from build123d import *

# Parameters (mm, degrees)
SKETCH1_R                = 2.55
BOSS_EXTRUDE1_DEPTH      = 5
SKETCH4_R                = 4.5
CUT_EXTRUDE2_DEPTH       = 1
SKETCH6_W                = 5.947651005
SKETCH6_H                = 20
BOSS_EXTRUDE2_DEPTH      = 4
BOSS_EXTRUDE2_DEPTH_BACK = 4
SKETCH11_R               = 4.5
CUT_EXTRUDE3_DEPTH       = 0.5
SKETCH16_R               = 3.25
BOSS_EXTRUDE3_DEPTH      = 3
BOSS_EXTRUDE3_DEPTH_BACK = 3
FILLET3_R                = 2
BOSS_EXTRUDE4_DEPTH      = 5.947651
CUT_EXTRUDE5_REACH       = 85
SKETCH18_R               = 3.25


with BuildPart() as part:
    # Sketch1 → Boss-Extrude1 (new body)
    with BuildSketch(Plane.XY):
        with BuildLine():
            Line((100, 25), (100, 20))
            ThreePointArc((100, 20), (99.414213562, 18.585786438), (98, 18))
            Line((98, 18), (72.248595461, 18))
            ThreePointArc((72.248595461, 18), (71.130561473, 17.658312395), (70.39454584, 16.75))
            ThreePointArc((70.39454584, 16.75), (50, 3), (29.60545416, 16.75))
            ThreePointArc((29.60545416, 16.75), (28.869438527, 17.658312395), (27.751404539, 18))
            Line((27.751404539, 18), (2, 18))
            ThreePointArc((2, 18), (0.585786438, 18.585786438), (0, 20))
            Line((0, 20), (0, 25))
            Line((0, 25), (0, 30))
            ThreePointArc((0, 30), (0.585786438, 31.414213562), (2, 32))
            Line((2, 32), (21.056240945, 32))
            Line((21.056240945, 32), (27.751404539, 32))
            ThreePointArc((27.751404539, 32), (28.869438527, 32.341687605), (29.60545416, 33.25))
            ThreePointArc((29.60545416, 33.25), (30.166752838, 34.520625347), (30.807119991, 35.753295167))
            ThreePointArc((30.807119991, 35.753295167), (32.106461975, 36.725482012), (33.699080137, 36.414026968))
            Line((33.699080137, 36.414026968), (35.34656276, 35.260447216))
            ThreePointArc((35.34656276, 35.260447216), (36.146649881, 34.078494315), (35.955031011, 32.664127224))
            ThreePointArc((35.955031011, 32.664127224), (50, 9), (64.044968989, 32.664127224))
            ThreePointArc((64.044968989, 32.664127224), (63.853350119, 34.078494315), (64.65343724, 35.260447216))
            Line((64.65343724, 35.260447216), (66.300919863, 36.414026968))
            ThreePointArc((66.300919863, 36.414026968), (67.893538025, 36.725482012), (69.192880009, 35.753295167))
            ThreePointArc((69.192880009, 35.753295167), (69.833247162, 34.520625347), (70.39454584, 33.25))
            ThreePointArc((70.39454584, 33.25), (71.130561473, 32.341687605), (72.248595461, 32))
            Line((72.248595461, 32), (78.943759055, 32))
            Line((78.943759055, 32), (98, 32))
            ThreePointArc((98, 32), (99.414213562, 31.414213562), (100, 30))
            Line((100, 30), (100, 25))
        make_face()
        with Locations((93, 25)):
            Circle(SKETCH1_R, mode=Mode.SUBTRACT)
        with Locations((7, 25)):
            Circle(SKETCH1_R, mode=Mode.SUBTRACT)
    extrude(amount=BOSS_EXTRUDE1_DEPTH)

    # Sketch4 → Cut-Extrude2 (cut)
    with BuildSketch(Plane.XY.offset(5)):
        with Locations((93, 25)):
            Circle(SKETCH4_R)
        with Locations((7, 25)):
            Circle(SKETCH4_R)
    extrude(amount=-CUT_EXTRUDE2_DEPTH, mode=Mode.SUBTRACT)

    # Sketch6 → Boss-Extrude2 (add, two sides)
    with BuildSketch(Plane(origin=(0, 25, 0), x_dir=(-1, 0, 0), z_dir=(0, -1, 0))) as boss_extrude2_sk:
        with Locations((-80.026174497, -15)):
            Rectangle(SKETCH6_W, SKETCH6_H)
    extrude(amount=BOSS_EXTRUDE2_DEPTH)
    extrude(boss_extrude2_sk.sketch, amount=-BOSS_EXTRUDE2_DEPTH_BACK)

    # Sketch11 → Cut-Extrude3 (cut)
    with BuildSketch(Plane(origin=(0, 0, 0), x_dir=(-1, 0, 0), z_dir=(0, 0, -1))):
        with Locations((-93, 25)):
            Circle(SKETCH11_R)
        with Locations((-7, 25)):
            Circle(SKETCH11_R)
    extrude(amount=-CUT_EXTRUDE3_DEPTH, mode=Mode.SUBTRACT)

    # Sketch16 → Boss-Extrude3 (add, two sides)
    with BuildSketch(Plane(origin=(0, 25, 0), x_dir=(-1, 0, 0), z_dir=(0, -1, 0))) as boss_extrude3_sk:
        with BuildLine():
            Line((-31.525983958, -5), (-31.525983958, -48.851508305))
            Line((-31.525983958, -48.851508305), (-31.525983958, -61))
            ThreePointArc((-31.525983958, -61), (-32.697556833, -63.828427125), (-35.525983958, -65))
            Line((-35.525983958, -65), (-43.054928699, -65))
            ThreePointArc((-43.054928699, -65), (-45.245818929, -64.346640106), (-46.720989255, -62.6))
            ThreePointArc((-46.720989255, -62.6), (-55.461014998, -59.950609847), (-56.692216044, -69))
            ThreePointArc((-56.692216044, -69), (-55.461014998, -78.049390153), (-46.720989255, -75.4))
            ThreePointArc((-46.720989255, -75.4), (-45.245818929, -73.653359894), (-43.054928699, -73))
            Line((-43.054928699, -73), (-25.956550891, -73))
            ThreePointArc((-25.956550891, -73), (-24.188489968, -71.525548017), (-23.525983958, -69.320750097))
            Line((-23.525983958, -69.320750097), (-23.525983958, -5))
            Line((-23.525983958, -5), (-31.525983958, -5))
        make_face()
        with Locations((-52.220080089, -73)):
            Circle(SKETCH16_R, mode=Mode.SUBTRACT)
        with Locations((-52.220080089, -65)):
            Circle(SKETCH16_R, mode=Mode.SUBTRACT)
    extrude(amount=BOSS_EXTRUDE3_DEPTH)
    extrude(boss_extrude3_sk.sketch, amount=-BOSS_EXTRUDE3_DEPTH_BACK)

    # Fillet3
    fillet3_edges = [part.edges().sort_by_distance(p)[0] for p in [
        (83, 25, 5),
        (80.026174498, 29, 5),
        (77.052348995, 25, 5),
        (80.026174498, 21, 5),
        (31.525983958, 25, 5),
        (27.525983958, 28, 5),
        (23.525983958, 25, 5),
        (27.525983958, 22, 5),
    ]]
    fillet(fillet3_edges, radius=FILLET3_R)

    # Sketch17 → Boss-Extrude4 (add)
    with BuildSketch(Plane(origin=(83, 0, 0), x_dir=(0, 0, -1), z_dir=(1, 0, 0))):
        with BuildLine():
            ThreePointArc((-19.547210182, 27.503414308), (-31, 25), (-19.547210182, 22.496585692))
            ThreePointArc((-19.547210182, 22.496585692), (-8.094420363, 25), (-19.547210182, 27.503414308))
        make_face()
    extrude(amount=-BOSS_EXTRUDE4_DEPTH)

    # Sketch18 → Cut-Extrude5 (cut, up to next)
    with BuildSketch(Plane(origin=(83, 0, 0), x_dir=(0, 0, -1), z_dir=(1, 0, 0)), mode=Mode.PRIVATE) as cut_extrude5_sk1:
        with Locations((-25, 25)):
            Circle(SKETCH18_R)
    cut_extrude5_tool1 = extrude(cut_extrude5_sk1.sketch, amount=-CUT_EXTRUDE5_REACH, mode=Mode.PRIVATE) & part.part
    add(cut_extrude5_tool1.solids().sort_by_distance((83, 25, 25))[0], mode=Mode.SUBTRACT)
    # Sketch18 → Cut-Extrude5 (cut, up to next)
    with BuildSketch(Plane(origin=(83, 0, 0), x_dir=(0, 0, -1), z_dir=(1, 0, 0)), mode=Mode.PRIVATE) as cut_extrude5_sk2:
        with Locations((-14.094420363, 25)):
            Circle(SKETCH18_R)
    cut_extrude5_tool2 = extrude(cut_extrude5_sk2.sketch, amount=-CUT_EXTRUDE5_REACH, mode=Mode.PRIVATE) & part.part
    add(cut_extrude5_tool2.solids().sort_by_distance((83, 25, 14.09442))[0], mode=Mode.SUBTRACT)


solid = part.part
Work out the finished part from the listing and answer in its coordinate system (mm). A direction names the side the tool comes from. Coordinates: 2 decimals unless noted, no trailing zeros. Write each loop counter-clockwise with the first axis right and the second up, starting at its lowest first coordinate (ties: lowest second). Pieces come first, ordered by that corner, then holes. Notation, with made-up numbers: M -5.75,-21 L 52.25,-21 A30 cw 52.25,5 Z; hole C 34,-12 d7. An arc over 180 degrees is marked long. Answer as CSV lines item,"result". Start each with the question number.
Item 1: Flat-ended cylindrical pins translate along their axes: P1, Ø2, axis at y = 22, z = 20.5, coming from the +X side; P2, Ø5, axis at y = 27, z = 33.5, coming from the -X side; P3, Ø10, axis at x = 7, y = 26.5, coming from the +Z side. Find the tip coordinate at first contact, or state that the pin passes through.
Item 2: A tool of negligible diameter and unlimited length cuts with its end or side. For faces 1 (the face through (80.07, 23.02, 16.67)), 2 (the face through (32.67, 24.96, 63.8)), 3 (the face through (85, 18, 2)), 4 (the face through (77.052, 25, 19)), 5 (the face through (85, 32, 2)), from which of +Z, -Z, +X, -X, +Y, -Y can it reach the whole face along a straight path? Write none if from no direction.
Item 3: Section B-B on x = 7 is taken. Write down the section's boundary in (y, z), and give its area (4 significant figures).
Item 4: Determine the mould class of faces 6 (the face through (27.61, 28.6, 5.57)), 7 (the face through (91, 23, 0.5)), 8 (the face through (76.45, 25.08, 5.57)) for opening direction Y: released by +Y, released by -Y, zero draft, split by the parting line, or undercut.
Item 5: Section D-D on y = 25 is taken. Give the number of separate pieces and of enclosed holes in the cut face, and give its area (3 significant figures).
Item 6: Section A-A on z = 25 is taken. Write down the section's boundary in (x, y).
Item 7: Consider L1, parallel to X at y = 27.5, z = 19; L2, parallel to Z at x = 34.5, y = 18.5; L3, parallel to Y at x = 7, z = 1. Determine where each line is inside the solid, lowest interval first.
Item 8: Section C-C on z = 14.5 is taken. Write down the section's boundary in (x, y).
Checks:
1,P1,"stops at x = 83"
1,P2,"stops at x = 23.53"
1,P3,"stops at z = 5"
2,face 1,"+X"
2,face 2,"+Y, -Y"
2,face 3,"+Z, -Z, +X, -Y"
2,face 4,"+Z, +Y, -Y"
2,face 5,"+Z, -Z, +X, +Y"
3,outline,"M 18,0 L 20.5,0 L 20.5,0.5 L 22.45,0.5 L 22.45,4 L 20.5,4 L 20.5,5 L 18,5 Z; M 27.55,0.5 L 29.5,0.5 L 29.5,0 L 32,0 L 32,5 L 29.5,5 L 29.5,4 L 27.55,4 Z"
3,area,"38.65 mm²"
4,face 6,"released by +Y"
4,face 7,"undercut"
4,face 8,"zero draft"
5,separate pieces,"6"
5,enclosed holes,"2"
5,area,"1,160 mm²"
6,outline,"M 23.53,22 L 31.53,22 L 31.53,28 L 23.53,28 Z; M 77.05,19 L 83,19 L 83,21.75 L 77.05,21.75 Z; M 77.05,28.25 L 83,28.25 L 83,31 L 77.05,31 Z"
7,L1,"x = 23.53 to 31.53, 77.05 to 83"
7,L2,"z = 0 to 5"
7,L3,"y = 18 to 22.45, 27.55 to 32"
8,outline,"M 23.53,22 L 31.53,22 L 31.53,28 L 23.53,28 Z; M 77.05,19.01 L 83,19.01 L 83,21.78 L 77.05,21.78 Z; M 77.05,28.22 L 83,28.22 L 83,30.99 L 77.05,30.99 Z"
